Geometry: final body of the model. Coordinates: model frame, mm. Give positions to 0.01 mm unless a question says otherwise; leave off trailing zeros. Loops run counter-clockwise (first coordinate to the right, second up) from the corner with the lowest first, then second, coordinate; pieces in that order, holes last. Notation, with made-up numbers: (47.25, 16) -> (64.25, 16) arc R20 cw to (64.25, 28) -> close; hole circle Ø4 at (69, -39). An arc over 180 degrees is marked (long way). One line per question, with ' | ' between items. Start each with the question number.
Item 1: Material intervals for line 1 along Y through (x, z) = (-111, 2.6); line 2 along X through (y, z) = (-8, 1.9); line 3 along Y through (x, z) = (87.5, 2.6), sorted ascending. Write a range as [from, to].
Item 2: Pin query (flat end, axial travel): P1, Ø2.5, axis at x = 110.86, y = -71.18, coming from the -Z side. Return the tip coordinate at first contact, or that it passes through.
Item 3: Section A-A on y = -123.5. Return loops of the section in (x, z).
Item 4: Section B-B on x = -95. Return loops of the section in (y, z), then the cut area to 3 significant figures.
Item 5: Section C-C on z = 1.95. Give the number of separate pieces and of enclosed holes in the cut face, then the cut area to 3 significant figures.
from build123d import *

# Parameters (mm, degrees)
SKETCH1_W           = 276
SKETCH1_H           = 339
SKETCH1_R           = 2.05
SKETCH1_W_2         = 206
SKETCH1_H_2         = 269
BOSS_EXTRUDE1_DEPTH = 3


with BuildPart() as part:
    # Sketch1 → Boss-Extrude1 (new body)
    with BuildSketch(Plane.XY):
        Rectangle(SKETCH1_W, SKETCH1_H)
        with Locations((-110.860879207, 142.360879207)):
            Circle(SKETCH1_R, mode=Mode.SUBTRACT)
        with Locations((-55.430439603, 142.360879207)):
            Circle(SKETCH1_R, mode=Mode.SUBTRACT)
        with Locations((-110.860879207, 71.180439603)):
            Circle(SKETCH1_R, mode=Mode.SUBTRACT)
        with Locations(Location((-55.430439603, -142.360879207, 0), (0, 0, 180))):
            Circle(SKETCH1_R, mode=Mode.SUBTRACT)
        with Locations(Location((-110.860879207, -142.360879207, 0), (0, 0, 180))):
            Circle(SKETCH1_R, mode=Mode.SUBTRACT)
        with Locations(Location((-110.860879207, -71.180439603, 0), (0, 0, 180))):
            Circle(SKETCH1_R, mode=Mode.SUBTRACT)
        with Locations(Location((55.430439603, 142.360879207, 0), (0, 0, 180))):
            Circle(SKETCH1_R, mode=Mode.SUBTRACT)
        with Locations(Location((110.860879207, 142.360879207, 0), (0, 0, 180))):
            Circle(SKETCH1_R, mode=Mode.SUBTRACT)
        with Locations(Location((110.860879207, 71.180439603, 0), (0, 0, 180))):
            Circle(SKETCH1_R, mode=Mode.SUBTRACT)
        with Locations((55.430439603, -142.360879207)):
            Circle(SKETCH1_R, mode=Mode.SUBTRACT)
        with Locations((110.860879207, -142.360879207)):
            Circle(SKETCH1_R, mode=Mode.SUBTRACT)
        with Locations((110.860879207, -71.180439603)):
            Circle(SKETCH1_R, mode=Mode.SUBTRACT)
        with Locations((-110.860879207, 0)):
            Circle(SKETCH1_R, mode=Mode.SUBTRACT)
        with Locations(Location((110.860879207, 0, 0), (0, 0, 180))):
            Circle(SKETCH1_R, mode=Mode.SUBTRACT)
        with Locations((0, 142.360879207)):
            Circle(SKETCH1_R, mode=Mode.SUBTRACT)
        with Locations(Location((0, -142.360879207, 0), (0, 0, 180))):
            Circle(SKETCH1_R, mode=Mode.SUBTRACT)
        Rectangle(SKETCH1_W_2, SKETCH1_H_2, mode=Mode.SUBTRACT)
    extrude(amount=BOSS_EXTRUDE1_DEPTH)


solid = part.part
Result sheet:
1) line 1: y = [-169.5, -144.41], [-140.32, -73.23], [-69.14, -2.05], [2.05, 69.14], [73.23, 140.32], [144.41, 169.5] | line 2: x = [-138, -103], [103, 138] | line 3: y = [-169.5, -134.5], [134.5, 169.5]
2) P1: passes through
3) outline: (-138, 0) -> (-103, 0) -> (-103, 3) -> (-138, 3) -> close; (103, 0) -> (138, 0) -> (138, 3) -> (103, 3) -> close
4) outline: (-169.5, 0) -> (-134.5, 0) -> (-134.5, 3) -> (-169.5, 3) -> close; (134.5, 0) -> (169.5, 0) -> (169.5, 3) -> (134.5, 3) -> close | area: 210 mm²
5) separate pieces: 1 | enclosed holes: 17 | area: 37,900 mm²
